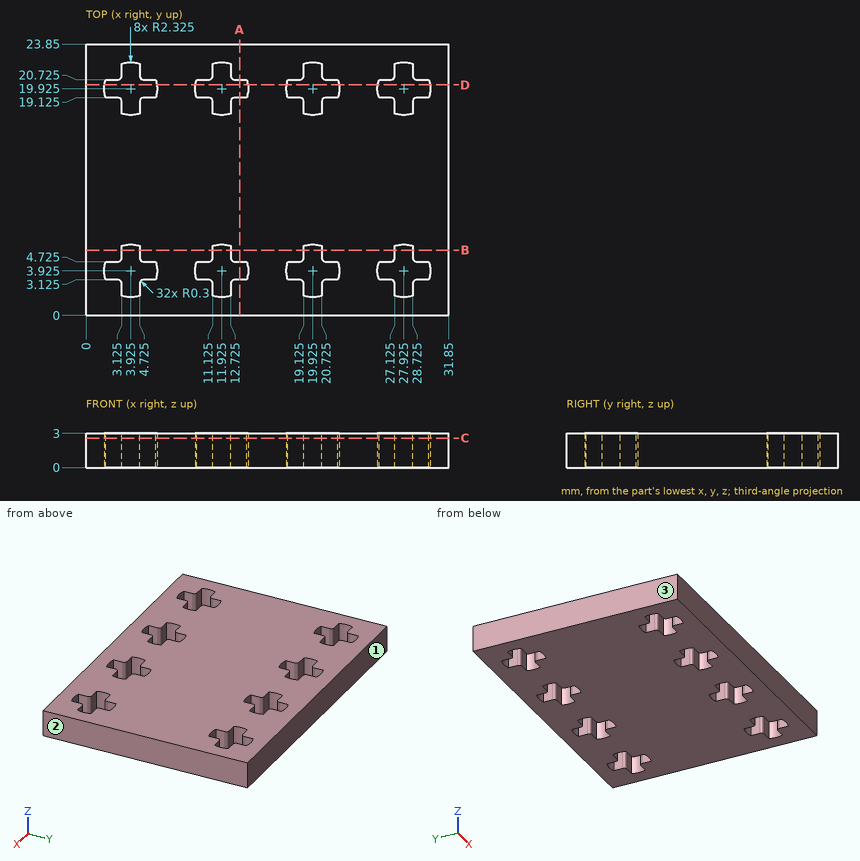
Could you check a few things on this drawing? It's one solid part, dimensions in mm from its lowest x, y, z. Coordinates: 2 decimals unless noted, no trailing zeros. Order: outer loops, then holes, each group sorted by start corner. A loop starts at its lowest first (then second) coordinate and runs counter-clockwise, first axis right, second up. Notation, with made-up numbers: (21, 34) -> (73, 34) arc R20 ccw to (73, 65) -> close; hole circle Ø10 at (75.5, -34). An arc over 180 degrees is marked (long way). One line per item, written item: value. Start each with the question number.
1) Imagine slicing it at D-D on y = 20.25. List the corners of the cut face in (x, z) for me.
2) Imagine slicing it at C-C on z = 2.6. Count the separate pieces of the cut face and the enclosed holes in it, plus the area to 3 significant figures.
3) If I drill on L1, parallel to X at y = 5, z = 1.65; L2, parallel to Y at x = 2.5, z = 2.55 (3 decimals); L3, parallel to Y at x = 4, z = 2.75, over which ranges is the centre line in solid material (lowest first)? Write a range as [from, to].
4) Imagine slicing it at A-A on x = 13.5. List the corners of the cut face in (y, z) for me (3 decimals).
5) We'd pull the mould along X, two halves only. Please class the marked faces 1, 2 and 3: +X half, -X half, draft (parallel to the pull), parting line (faces both ways), or undercut.
6) Imagine slicing it at B-B on y = 5.75. List the corners of the cut face in (x, z) for me (3 decimals).
Answer list:
1. outline: (0, 0) -> (1.62, 0) -> (1.62, 3) -> (0, 3) -> close; (6.23, 0) -> (9.62, 0) -> (9.62, 3) -> (6.23, 3) -> close; (14.23, 0) -> (17.62, 0) -> (17.62, 3) -> (14.23, 3) -> close; (22.23, 0) -> (25.62, 0) -> (25.62, 3) -> (22.23, 3) -> close; (30.23, 0) -> (31.85, 0) -> (31.85, 3) -> (30.23, 3) -> close
2. separate pieces: 1
2. enclosed holes: 8
2. area: 663 mm2
3. L1: x = [0, 3.12], [4.73, 11.12], [12.73, 19.12], [20.73, 27.12], [28.73, 31.85]
3. L2: y = [0, 3.125], [4.725, 19.125], [20.725, 23.85]
3. L3: y = [0, 1.6], [6.25, 17.6], [22.25, 23.85]
4. outline: (0, 0) -> (3.125, 0) -> (3.125, 3) -> (0, 3) -> close; (4.725, 0) -> (19.125, 0) -> (19.125, 3) -> (4.725, 3) -> close; (20.725, 0) -> (23.85, 0) -> (23.85, 3) -> (20.725, 3) -> close
5. face 1: draft
5. face 2: +X half
5. face 3: -X half
6. outline: (0, 0) -> (3.125, 0) -> (3.125, 3) -> (0, 3) -> close; (4.725, 0) -> (11.125, 0) -> (11.125, 3) -> (4.725, 3) -> close; (12.725, 0) -> (19.125, 0) -> (19.125, 3) -> (12.725, 3) -> close; (20.725, 0) -> (27.125, 0) -> (27.125, 3) -> (20.725, 3) -> close; (28.725, 0) -> (31.85, 0) -> (31.85, 3) -> (28.725, 3) -> close
